Verification items for the finished model (mm, model axes). Face numbers are marked on the shaded views. A direction names the side the tool comes from. Round coordinates to 2 decimals unless told otherwise and drop trailing zeros. Order: outer loops, then holes, each group sorted by start corner. A loop starts at its lowest first (then second) coordinate and runs counter-clockwise, first axis right, second up. Notation, with made-up numbers: M 41.25,35 L 87.25,35 A19 cw 87.25,56 Z; hole C 49,49.25 d7. An arc over 180 degrees is marked long. Write item = value, one per line. Start each with the question number.
from build123d import *

# Parameters (mm, degrees)
SKETCH_1_R      = 30
SKETCH_1_R_2    = 4.5
EXTRUDE_2_DEPTH = 10
SKETCH_3_R      = 4.5
SKETCH_3_R_2    = 2.5
EXTRUDE_3_DEPTH = 3
FILLET_1_R      = 1


with BuildPart() as part:
    # ｽｹｯﾁ1 → ﾎﾞｽ - 押し出し2 (new body)
    with BuildSketch(Plane(origin=(0, 0, 0), x_dir=(1, 0, 0), z_dir=(0, 1, 0))):
        Circle(SKETCH_1_R)
        with Locations((0, -22.65)):
            Circle(SKETCH_1_R_2, mode=Mode.SUBTRACT)
        with Locations((-19.615475396, -11.325)):
            Circle(SKETCH_1_R_2, mode=Mode.SUBTRACT)
        with Locations((-19.615475396, 11.325)):
            Circle(SKETCH_1_R_2, mode=Mode.SUBTRACT)
        with Locations((0, 22.65)):
            Circle(SKETCH_1_R_2, mode=Mode.SUBTRACT)
        with Locations((19.615475396, 11.325)):
            Circle(SKETCH_1_R_2, mode=Mode.SUBTRACT)
        with Locations((19.615475396, -11.325)):
            Circle(SKETCH_1_R_2, mode=Mode.SUBTRACT)
    extrude(amount=EXTRUDE_2_DEPTH)

    # ｽｹｯﾁ3 → ﾎﾞｽ - 押し出し3 (add)
    with BuildSketch(Plane.XZ):
        with Locations((-19.615475396, -11.325)):
            Circle(SKETCH_3_R)
        with Locations((-19.615475396, -11.325)):
            Circle(SKETCH_3_R_2, mode=Mode.SUBTRACT)
        with Locations((-19.615475396, 11.325)):
            Circle(SKETCH_3_R)
        with Locations((-19.615475396, 11.325)):
            Circle(SKETCH_3_R_2, mode=Mode.SUBTRACT)
        with Locations((0, 22.65)):
            Circle(SKETCH_3_R)
        with Locations((0, 22.65)):
            Circle(SKETCH_3_R_2, mode=Mode.SUBTRACT)
        with Locations((19.615475396, 11.325)):
            Circle(SKETCH_3_R)
        with Locations((19.615475396, 11.325)):
            Circle(SKETCH_3_R_2, mode=Mode.SUBTRACT)
        with Locations((19.615475396, -11.325)):
            Circle(SKETCH_3_R)
        with Locations((19.615475396, -11.325)):
            Circle(SKETCH_3_R_2, mode=Mode.SUBTRACT)
        with Locations((0, -22.65)):
            Circle(SKETCH_3_R)
        with Locations((0, -22.65)):
            Circle(SKETCH_3_R_2, mode=Mode.SUBTRACT)
    extrude(amount=-EXTRUDE_3_DEPTH)

    # ﾌｨﾚｯﾄ1
    fillet_1_edges = [part.edges().sort_by_distance(p)[0] for p in [
        (-30, 10, 0),
    ]]
    fillet(fillet_1_edges, radius=FILLET_1_R)


solid = part.part
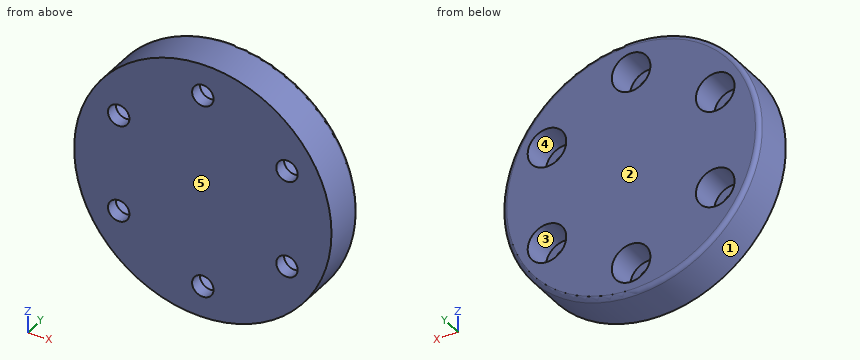
1) Cross-section at B-B, the plane z = -10. Give the number of separate pieces and of enclosed holes in the cut face, then the cut area to 3 significant figures.
2) Scan lines: probe 1 along Z at (x, y) = (0.5, 3.5); probe 2 along Z at (x, y) = (-16, 5.25); probe 3 along X at (y, z) = (4.5, -14). Record each from-to range of solid material in increasing order.
3) Cross-section at A-A, the plane x = 0. Enter the section's corners in (y, z).
4) Release check for a two-part mould opening along X. For the marked faces 1, 2 and 3 record: pulls with the +X half, pulls with the -X half, needs draft (parallel to the pull), parting line crosses it, or undercut.
5) Gauge pin test, flat ends, axial feed: P1, Ø4, axis at x = -15, y = 8.5, coming from the +Z side; P2, Ø2.5, axis at x = -1.5, z = -22, coming from the +Y side; P3, Ø6, axis at y = 2.5, z = 6, coming from the -X side. Record the tip position at first contact, or that the pin passes through.
6) Access from +Z, -Z, +X, -X, +Y, -Y to the whole of each face (thin tool, end or side, straight path). Record for the marked faces 4 and 5.
Geometry results:
q1.separate_pieces = 3
q1.enclosed_holes = 0
q1.area = 419 mm^2
q2.probe_1 = -30 to -27.12, -18.18 to 18.18, 27.12 to 30
q2.probe_2 = -25.38 to -14, -8.65 to 8.65, 14 to 25.38
q2.probe_3 = -26.53 to -23.23, -16 to 16, 23.23 to 26.53
q3.outline = M 0,-30 L 9,-30 A1 ccw 10,-29 L 10,-27.15 L 3,-27.15 L 3,-25.15 L 0,-25.15 Z; M 0,-20.15 L 3,-20.15 L 3,-18.15 L 10,-18.15 L 10,18.15 L 3,18.15 L 3,20.15 L 0,20.15 Z; M 0,25.15 L 3,25.15 L 3,27.15 L 10,27.15 L 10,29 A1 ccw 9,30 L 0,30 Z
q4.face_1 = parting line crosses it
q4.face_2 = needs draft
q4.face_3 = undercut
q5.P1 = 27.04
q5.P2 = 3
q5.P3 = -29.85
q6.face_4 = +Y
q6.face_5 = +Z, -Z, +X, -X, -Y
